For this review, take the finished solid that the model builds, in its own axes (mm). A direction names the side the tool comes from. Coordinates: 2 decimals unless noted, no trailing zeros. Loops run counter-clockwise (first coordinate to the right, second up) from the corner with the lowest first, then second, coordinate; pieces in that order, holes last. Notation, with made-up numbers: (11.25, 0.25) - (54.25, 0.25) arc R27 cw to (54.25, 38.25) - close; hole circle Ø6 at (-33.75, 16.5). An arc over 180 degrees is marked (long way). Answer as a JSON object with one key per item and string values. Group by question number.
Item 1: Clearance check with flat-ended pins moving along their axes: pin 1 (0.8 mm diameter, centred on y = -7, z = 6, fed in from -X); pin 2 (1.9 mm diameter, centred on x = -2, y = -8, fed in from -Z); pin 3 (1.6 mm diameter, centred on x = 1, y = 1, fed in from -Z). State where each tip first meets the part, or that it passes through.
Item 2: We need section C-C (y = -2.25). Give the boundary of the cut face in (x, z), then the cut area to 3 significant figures.
Item 3: We need section D-D (z = -3). Give the boundary of the cut face in (x, y) (3 decimals).
Item 4: Tool access review of faces 1 (the flat face through (-23, -6, -6)), 2 (the flat face through (0, -6, 7.144)), 3 (the flat face through (0, 3.175, -1)), 4 (the flat face through (0, 0, 3)), 5 (the flat face through (21, -9.525, 0)): name each direction out of +Z, -Z, +X, -X, +Y, -Y from which nothing blocks a thin tool from reaching the whole face with its end or side.
Item 5: To check wall thickness, follow line 1 (Z direction, x = 9, y = -4); line 2 (Z direction, x = 27, y = 1.25); line 3 (Z direction, x = -10, y = -1.9). State the ranges of each line that lie inside material, in increasing order.
Item 6: Mouldability with a two-part tool opening along X and no side actions: class faces 6 (the flat face through (23, -6, -6)), 7 (the cylindrical face through (-11.25, -1.61, 0.05)), 8 (the cylindrical face through (24, 2, -8)), 9 (the flat face through (-26, 3.175, 7)) as released by +X, released by -X, zero draft, split by the parting line, or undercut.
Item 7: We need section A-A (x = -10). Give the boundary of the cut face in (y, z) (3 decimals).
Item 8: We need section B-B (z = 0). Give the boundary of the cut face in (x, y) (3 decimals), then the cut area to 3 significant figures.
from build123d import *

# Parameters (mm, degrees)
F1_DEPTH = 9.525
F2_W     = 19
F2_H     = 1.5875
F2_W_2   = 62
F4_DEPTH = 6.35
F5_R     = 3
F5_R_2   = 1.25
F5_W     = 4.6
F5_H     = 6.1
F7_DEPTH = 6.35
F5_W_2   = 8
F5_H_2   = 7
F5_W_3   = 4
F5_H_3   = 4
F8_DEPTH = 6.351
F9_DEPTH = 6.351


with BuildPart() as f1:
    # F0 (on Front) → F1 (new body)
    with BuildSketch(Plane.XZ):
        Polygon((-12, 13.4935), (-31, 13.4935), (-31, -13.4935), (-12, -13.4935), (-12, -10.31875), (0, -10.31875), (12, -10.31875), (12, -13.4935), (31, -13.4935), (31, 13.4935), (12, 13.4935), (12, 10.31875), (0, 10.31875), (-12, 10.31875), align=None)
    extrude(amount=F1_DEPTH)

    # F2 (on face) → F4 (cut, through all)
    with BuildSketch(Plane.XZ.offset(9.525)):
        with Locations((-21.5, 11.1125)):
            Rectangle(F2_W, F2_H)
        with Locations((21.5, 11.1125)):
            Rectangle(F2_W, F2_H)
        with Locations((0, 7.9375)):
            Rectangle(F2_W_2, F2_H)
        with Locations((0, 4.7625)):
            Rectangle(F2_W_2, F2_H)
        with Locations((0, 1.5875)):
            Rectangle(F2_W_2, F2_H)
        with Locations((0, -1.5875)):
            Rectangle(F2_W_2, F2_H)
        with Locations((0, -4.7625)):
            Rectangle(F2_W_2, F2_H)
        with Locations((0, -7.9375)):
            Rectangle(F2_W_2, F2_H)
        with Locations((-21.5, -11.1125)):
            Rectangle(F2_W, F2_H)
        with Locations((21.5, -11.1125)):
            Rectangle(F2_W, F2_H)
    extrude(amount=-F4_DEPTH, mode=Mode.SUBTRACT)

    # F5 (on offset) → F7 (join, through all)
    with BuildSketch(Plane.XZ.offset(3.175)):
        with Locations((-27, 8)):
            Circle(F5_R)
        with Locations((-27, 8)):
            Circle(F5_R_2, mode=Mode.SUBTRACT)
        with Locations((-27, -8)):
            Circle(F5_R)
        with Locations((-27, -8)):
            Circle(F5_R_2, mode=Mode.SUBTRACT)
        with Locations((27, 8)):
            Circle(F5_R)
        with Locations((27, 8)):
            Circle(F5_R_2, mode=Mode.SUBTRACT)
        with Locations((27, -8)):
            Circle(F5_R)
        with Locations((27, -8)):
            Circle(F5_R_2, mode=Mode.SUBTRACT)
        with Locations((0, -1.25)):
            Rectangle(F5_W, F5_H)
    extrude(amount=-F7_DEPTH)

    # F5 (on offset) → F8 (cut, through all)
    with BuildSketch(Plane.XZ.offset(3.175)):
        with Locations((-27, 8)):
            Rectangle(F5_W_2, F5_H_2)
        with Locations((-27, 8)):
            Circle(F5_R, mode=Mode.SUBTRACT)
        with Locations((-27, -8)):
            Rectangle(F5_W_2, F5_H_2)
        with Locations((-27, -8)):
            Circle(F5_R, mode=Mode.SUBTRACT)
        with Locations((27, 8)):
            Rectangle(F5_W_2, F5_H_2)
        with Locations((27, 8)):
            Circle(F5_R, mode=Mode.SUBTRACT)
        with Locations((27, -8)):
            Rectangle(F5_W_2, F5_H_2)
        with Locations((27, -8)):
            Circle(F5_R, mode=Mode.SUBTRACT)
        with Locations((-27, 8)):
            Circle(F5_R)
        with Locations((-27, 8)):
            Circle(F5_R_2, mode=Mode.SUBTRACT)
        with Locations((-27, -8)):
            Circle(F5_R)
        with Locations((-27, -8)):
            Circle(F5_R_2, mode=Mode.SUBTRACT)
        with Locations((27, 8)):
            Circle(F5_R)
        with Locations((27, 8)):
            Circle(F5_R_2, mode=Mode.SUBTRACT)
        with Locations((27, -8)):
            Circle(F5_R)
        with Locations((27, -8)):
            Circle(F5_R_2, mode=Mode.SUBTRACT)
        with Locations((-10, 0)):
            Rectangle(F5_W_3, F5_H_3)
        with Locations((-10, 0)):
            Circle(F5_R_2, mode=Mode.SUBTRACT)
        with Locations((10, 0)):
            Rectangle(F5_W_3, F5_H_3)
        with Locations((10, 0)):
            Circle(F5_R_2, mode=Mode.SUBTRACT)
        with Locations((-27, 8)):
            Circle(F5_R_2)
        with Locations((-27, -8)):
            Circle(F5_R_2)
        with Locations((-10, 0)):
            Circle(F5_R_2)
        with Locations((27, 8)):
            Circle(F5_R_2)
        with Locations((27, -8)):
            Circle(F5_R_2)
        with Locations((10, 0)):
            Circle(F5_R_2)
    extrude(amount=F8_DEPTH, mode=Mode.SUBTRACT)

    # F5 (on offset) → F9 (cut, through all)
    with BuildSketch(Plane.XZ.offset(3.175)):
        with Locations((-27, 8)):
            Circle(F5_R_2)
        with Locations((-27, -8)):
            Circle(F5_R_2)
        with Locations((27, 8)):
            Circle(F5_R_2)
        with Locations((27, -8)):
            Circle(F5_R_2)
        with Locations((-10, 0)):
            Circle(F5_R_2)
        with Locations((10, 0)):
            Circle(F5_R_2)
    extrude(amount=-F9_DEPTH, mode=Mode.SUBTRACT)


solid = f1.part
Check sheet entries:
{
 "1": {"pin 1": "stops at x = -23", "pin 2": "stops at z = -10.32", "pin 3": "stops at z = -4.3"},
 "2": {"outline": "(-31, -13.49) - (-12, -13.49) - (-12, -10.32) - (12, -10.32) - (12, -13.49) - (31, -13.49) - (31, 13.49) - (12, 13.49) - (12, 10.32) - (-12, 10.32) - (-12, 13.49) - (-31, 13.49) - close; hole circle Ø2.5 at (-27, -8); hole circle Ø2.5 at (-27, 8); hole circle Ø2.5 at (-10, 0); hole circle Ø2.5 at (10, 0); hole circle Ø2.5 at (27, -8); hole circle Ø2.5 at (27, 8)", "area": "1,490 mm2"},
 "3": {"outline": "(-31, -9.525) - (31, -9.525) - (31, 0) - (2.3, 0) - (2.3, 3.175) - (-2.3, 3.175) - (-2.3, 0) - (-31, 0) - close"},
 "4": {"face 1": "-X, -Y", "face 2": "+X, -X, -Y", "face 3": "+Z, -Z, +X, -X, +Y", "face 4": "+Y", "face 5": "+Z, -Z, +X, -X, -Y"},
 "5": {"line 1": "z = -10.32 to -8.73, -7.14 to -5.56, -3.97 to -2.38, 2.38 to 3.97, 5.56 to 7.14, 8.73 to 10.32", "line 2": "z = -11 to -9.25, -6.75 to -5, 5 to 6.75, 9.25 to 11", "line 3": "z = -10.32 to -1.25, 1.25 to 10.32"},
 "6": {"face 6": "released by +X", "face 7": "undercut", "face 8": "undercut", "face 9": "zero draft"},
 "7": {"outline": "(-9.525, -10.319) - (0, -10.319) - (0, -1.25) - (-3.175, -1.25) - (-3.175, -2.381) - (-9.525, -2.381) - (-9.525, -3.969) - (-3.175, -3.969) - (-3.175, -5.556) - (-9.525, -5.556) - (-9.525, -7.144) - (-3.175, -7.144) - (-3.175, -8.731) - (-9.525, -8.731) - close; (-9.525, 2.381) - (-3.175, 2.381) - (-3.175, 1.25) - (0, 1.25) - (0, 10.319) - (-9.525, 10.319) - (-9.525, 8.731) - (-3.175, 8.731) - (-3.175, 7.144) - (-9.525, 7.144) - (-9.525, 5.556) - (-3.175, 5.556) - (-3.175, 3.969) - (-9.525, 3.969) - close"},
 "8": {"outline": "(-31, -9.525) - (-12, -9.525) - (-12, -3.175) - (-11.25, -3.175) - (-11.25, 0) - (-31, 0) - close; (-8.75, -3.175) - (-8, -3.175) - (-8, -9.525) - (8, -9.525) - (8, -3.175) - (8.75, -3.175) - (8.75, 0) - (2.3, 0) - (2.3, 3.175) - (-2.3, 3.175) - (-2.3, 0) - (-8.75, 0) - close; (11.25, -3.175) - (12, -3.175) - (12, -9.525) - (31, -9.525) - (31, 0) - (11.25, 0) - close", "area": "538 mm2"}
}
